Autodesk Inventor part; units mm, degrees
ref_plane "YZ Plane" through (0, 0, 0) normal (1, 0, 0) x (0, 1, 0)
ref_plane "XZ Plane" through (0, 0, 0) normal (0, 1, 0) x (-1, 0, 0)
ref_plane "XY Plane" through (0, 0, 0) normal (0, 0, 1) x (1, 0, 0)
sketch "Sketch1" plane through (0, 0, 0) normal (0, 0, 1) x (1, 0, 0)
  line L0 (-21, 5.5) -> (21, 5.5)
  line L1 (21, 5.5) -> (21, -5.5)
  line L2 (21, -5.5) -> (-21, -5.5)
  line L3 (-21, -5.5) -> (-21, 5.5)
  circle A0 centre (-15.5, 0) radius 1.6
  circle A1 centre (15.5, 0) radius 1.6
  point P0 (0, 0)
  point P1 (0, 5.5)
  point P2 (-21, 0)
  dimension "d0" = 31
  dimension "d1" = 15.5
  dimension "d2" = 5.5
  dimension "d3" = 5.5
  dimension "d4" = 3.2
extrude "Extrusion1" add sketch "Sketch1" along normal blind 4
sketch "Sketch2" plane through (-21, 5.5, 0) normal (0, 1, 0) x (1, 0, 0)
  circle A0 centre (24.25, -2) radius 0.4
  circle A1 centre (17.75, -2) radius 0.4
  line L0 (0, 0) -> (0, -4)
  point P0 (21, 0)
  point P1 (0, -2)
  dimension "d7" = 6.5
  dimension "d8" = 3.25
  dimension "d9" = 0.8
extrude "Extrusion2" cut sketch "Sketch2" against normal through all
properties part number "Endschalterhalter"
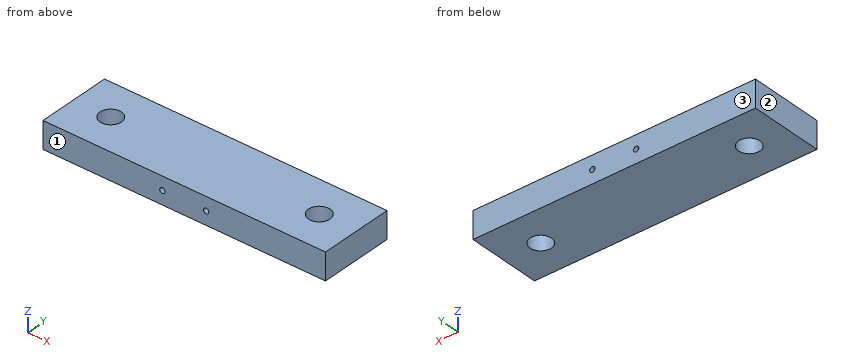
Design review of the part built by this model. Coordinates are the model's own, in mm. Face numbers are marked on the shaded views. Give positions to 0.01 mm unless a question says otherwise; leave off trailing zeros. Loops run counter-clockwise (first coordinate to the right, second up) from the corner with the lowest first, then second, coordinate; pieces in that order, holes last. Notation, with made-up numbers: (34.5, 39.25) -> (68.5, 39.25) arc R15 cw to (68.5, 49.25) -> close; hole circle Ø1 at (1, 88.25). An arc over 180 degrees is marked (long way). One line per question, with ' | ' between items. Start each with the question number.
(1) Insertion check: P1, Ø2.5, axis at x = 15.5, y = 0, coming from the -Z side. The pin has a flat end and moves straight along its axis. Give the tip position at first contact, or say it passes through.
(2) We need section B-B (z = 2). State the section outline as (x, y) points.
(3) For line 1 (Z direction, x = 3.25, y = -2); line 2 (X direction, y = -0.75, z = 3.25); line 3 (X direction, y = 1.25, z = 2.95), list the stretches that pass through material, from the lowest coordinate up.
(4) Draft analysis for pull direction Y (two halves, no side actions). For the marked faces 1, 2 and 3, state which applies: +Y half, -Y half, draft (parallel to the pull), parting line (faces both ways), or undercut.
(5) We need section A-A (x = -15.5). State the section outline as (y, z) points.
(6) We need section D-D (x = 3.25). State the section outline as (y, z) points, and give its area (3 significant figures).
(7) We need section C-C (y = -0.5). State the section outline as (x, z) points.
The answers:
1) P1: passes through
2) outline: (-21, -5.5) -> (-3.65, -5.5) -> (-3.65, 5.5) -> (-21, 5.5) -> close; (-2.85, -5.5) -> (2.85, -5.5) -> (2.85, 5.5) -> (-2.85, 5.5) -> close; (3.65, -5.5) -> (21, -5.5) -> (21, 5.5) -> (3.65, 5.5) -> close; hole circle Ø3.2 at (-15.5, 0); hole circle Ø3.2 at (15.5, 0)
3) line 1: z = 0 to 1.6, 2.4 to 4 | line 2: x = -21 to -16.91, -14.09 to 14.09, 16.91 to 21 | line 3: x = -21 to -16.5, -14.5 to 14.5, 16.5 to 21
4) face 1: -Y half | face 2: draft | face 3: +Y half
5) outline: (-5.5, 0) -> (-1.6, 0) -> (-1.6, 4) -> (-5.5, 4) -> close; (1.6, 0) -> (5.5, 0) -> (5.5, 4) -> (1.6, 4) -> close
6) outline: (-5.5, 0) -> (5.5, 0) -> (5.5, 1.6) -> (-5.5, 1.6) -> close; (-5.5, 2.4) -> (5.5, 2.4) -> (5.5, 4) -> (-5.5, 4) -> close | area: 35.2 mm^2
7) outline: (-21, 0) -> (-17.02, 0) -> (-17.02, 4) -> (-21, 4) -> close; (-13.98, 0) -> (13.98, 0) -> (13.98, 4) -> (-13.98, 4) -> close; (17.02, 0) -> (21, 0) -> (21, 4) -> (17.02, 4) -> close; hole circle Ø0.8 at (-3.25, 2); hole circle Ø0.8 at (3.25, 2)
